Geometry: final body of the model. Coordinates: model frame, mm. Coordinates: 2 decimals unless noted, no trailing zeros. Order: outer loops, then holes, each group sorted by start corner. A loop starts at its lowest first (then second) coordinate and runs counter-clockwise, first axis right, second up. Notation, with made-up numbers: (-30, -9.5) -> (12, -9.5) arc R21 ccw to (12, 3.5) -> close; hole circle Ø4 at (-14, 28.25). An arc over 180 degrees is marked (long way). Use one line per item in the form item = value.
```python
from build123d import *

# Parameters (mm, degrees)
SKETCH_1_R      = 33.5
SKETCH_1_R_2    = 12.7
SKETCH_1_R_3    = 1.4
SKETCH_1_R_4    = 2
EXTRUDE_1_DEPTH = 1


with BuildPart() as part:
    # 草图1 → 凸台-拉伸1 (new body)
    with BuildSketch(Plane.XY):
        Circle(SKETCH_1_R)
        Circle(SKETCH_1_R_2, mode=Mode.SUBTRACT)
        with Locations((0, -26.5)):
            Circle(SKETCH_1_R_3, mode=Mode.SUBTRACT)
        with Locations((-25.202997682, -8.188950351)):
            Circle(SKETCH_1_R_3, mode=Mode.SUBTRACT)
        with Locations((-15.576309186, 21.438950351)):
            Circle(SKETCH_1_R_3, mode=Mode.SUBTRACT)
        with Locations((15.576309186, 21.438950351)):
            Circle(SKETCH_1_R_3, mode=Mode.SUBTRACT)
        with Locations((25.202997682, -8.188950351)):
            Circle(SKETCH_1_R_3, mode=Mode.SUBTRACT)
        with Locations((-8.651773631, -26.627421273)):
            Circle(SKETCH_1_R_4, mode=Mode.SUBTRACT)
        with Locations(Location((8.651773631, -26.627421273, 0), (0, 0, 180))):
            Circle(SKETCH_1_R_4, mode=Mode.SUBTRACT)
        with Locations((-27.997727597, 0)):
            Circle(SKETCH_1_R_4, mode=Mode.SUBTRACT)
        with Locations(Location((-22.65063743, -16.456651379, 0), (0, 0, 180))):
            Circle(SKETCH_1_R_4, mode=Mode.SUBTRACT)
        with Locations((-8.651773631, 26.627421273)):
            Circle(SKETCH_1_R_4, mode=Mode.SUBTRACT)
        with Locations(Location((-22.65063743, 16.456651379, 0), (0, 0, 180))):
            Circle(SKETCH_1_R_4, mode=Mode.SUBTRACT)
        with Locations((22.65063743, 16.456651379)):
            Circle(SKETCH_1_R_4, mode=Mode.SUBTRACT)
        with Locations(Location((8.651773631, 26.627421273, 0), (0, 0, 180))):
            Circle(SKETCH_1_R_4, mode=Mode.SUBTRACT)
        with Locations((22.65063743, -16.456651379)):
            Circle(SKETCH_1_R_4, mode=Mode.SUBTRACT)
        with Locations(Location((27.997727597, 0, 0), (0, 0, 180))):
            Circle(SKETCH_1_R_4, mode=Mode.SUBTRACT)
        with BuildLine():
            Line((-19.308819678, -20.581224709), (-14.606537659, -14.109088754))
            ThreePointArc((-14.606537659, -14.109088754), (-9.684453912, -13.329507274), (-8.904872432, -18.251591021))
            Line((-8.904872432, -18.251591021), (-13.607154451, -24.723726976))
            ThreePointArc((-13.607154451, -24.723726976), (-18.529238198, -25.503308456), (-19.308819678, -20.581224709))
        make_face(mode=Mode.SUBTRACT)
        with BuildLine():
            Line((-25.540661294, 12.003830576), (-17.932209164, 9.531694621))
            ThreePointArc((-17.932209164, 9.531694621), (-15.669775592, 5.091418725), (-20.110051488, 2.828985154))
            Line((-20.110051488, 2.828985154), (-27.718503618, 5.301121109))
            ThreePointArc((-27.718503618, 5.301121109), (-29.98093719, 9.741397005), (-25.540661294, 12.003830576))
        make_face(mode=Mode.SUBTRACT)
        with BuildLine():
            Line((3.523822903, 28), (3.523822903, 20))
            ThreePointArc((3.523822903, 20), (0, 16.476177097), (-3.523822903, 20))
            Line((-3.523822903, 20), (-3.523822903, 28))
            ThreePointArc((-3.523822903, 28), (0, 31.523822903), (3.523822903, 28))
        make_face(mode=Mode.SUBTRACT)
        with BuildLine():
            Line((27.718503618, 5.301121109), (20.110051488, 2.828985154))
            ThreePointArc((20.110051488, 2.828985154), (15.669775592, 5.091418725), (17.932209164, 9.531694621))
            Line((17.932209164, 9.531694621), (25.540661294, 12.003830576))
            ThreePointArc((25.540661294, 12.003830576), (29.98093719, 9.741397005), (27.718503618, 5.301121109))
        make_face(mode=Mode.SUBTRACT)
        with BuildLine():
            Line((13.607154451, -24.723726976), (8.904872432, -18.251591021))
            ThreePointArc((8.904872432, -18.251591021), (9.684453912, -13.329507274), (14.606537659, -14.109088754))
            Line((14.606537659, -14.109088754), (19.308819678, -20.581224709))
            ThreePointArc((19.308819678, -20.581224709), (18.529238198, -25.503308456), (13.607154451, -24.723726976))
        make_face(mode=Mode.SUBTRACT)
    extrude(amount=EXTRUDE_1_DEPTH)


solid = part.part
```
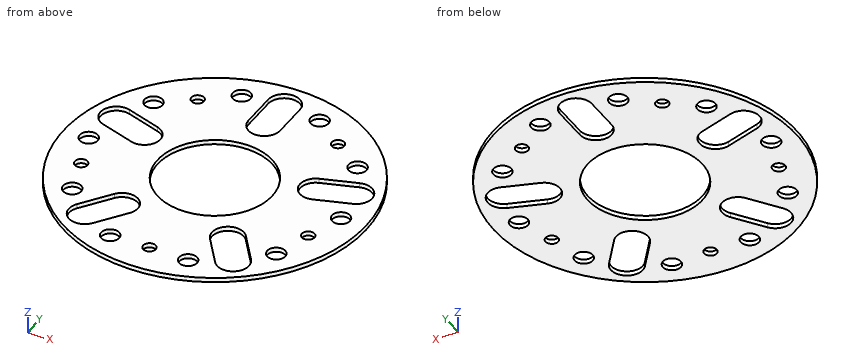
1) Material intervals for probe 1 along Y at (x, z) = (0, 0.4); probe 2 along Y at (x, z) = (-21, 0.5); probe 3 along X at (y, z) = (25.5, 0.9), sorted ascending. Write a range as from..to.
Results found:
probe_1 = -33.5..-27.9, -25.1..-12.7, 12.7..16.48, 31.52..33.5
probe_2 = -26.1..-17.59, -15.33..3.12, 10.53..15.33, 17.59..26.1
probe_3 = -21.73..-10.3, -7..-3.52, 3.52..7, 10.3..21.73
2) Section A-A, the plane y = 0. Output: boundary loops of the cut face in (x, z).
Results found:
outline = (-33.5, 0) -> (-30, 0) -> (-30, 1) -> (-33.5, 1) -> close; (-26, 0) -> (-12.7, 0) -> (-12.7, 1) -> (-26, 1) -> close; (12.7, 0) -> (26, 0) -> (26, 1) -> (12.7, 1) -> close; (30, 0) -> (33.5, 0) -> (33.5, 1) -> (30, 1) -> close
3) Section B-B, the plane z = 0.15. Give the number of separate pieces and of enclosed holes in the cut face, and give its area (3 significant figures).
Results found:
separate_pieces = 1
enclosed_holes = 21
area = 2,390 mm2
